Could you check a few things on this model? Use its own coordinates, in mm. A direction names the side the tool comes from. Coordinates: 2 decimals unless noted, no trailing zeros. Order: outer loops, then holes, each group sorted by start corner. A loop starts at its lowest first (then second) coordinate and runs counter-clockwise, first axis right, second up. Notation, with made-up numbers: (85, -32.75) -> (98, -32.75) arc R14 cw to (98, -25.75) -> close; hole circle Ø5 at (-31, -22.75). An arc over 180 degrees is marked (long way). Use a Markdown table: item, result. Add a question column.
1) Thinking about a two-plate mould opening in X: for faces 5 (the flat face through (2.54, 169, 0)), 6 (the flat face through (63, 75, 7.938)), 7 (the flat face through (20.4, 323.85, -0.1)), which applies, +X half, -X half, draft (parallel to the pull), parting line (faces both ways), or undercut?
2) If I drill on L1, parallel to X at y = 281, z = 2; L2, parallel to X at y = 40, z = 4 (1 decimal); L3, parallel to Y at x = 10, z = -2.5 (3 decimals), over which ranges is the centre line in solid material (lowest first)? Write a range as [from, to].
3) Will these pins go through, and if not, where does the flat tip stop? pin 1 Ø15 at (x, z) = (64, -2.5) entering from +Y; pin 2 Ø8 at (x, y) = (13, 140.5) entering from -Z (3 decimals); pin 3 Ø5 at (y, z) = (285.5, 10) entering from -X; pin 4 Ø15 at (x, y) = (63.5, 0) entering from -Z.
4) If we section it at A-A (y = 0): Write out the boundary of the cut face in (x, z) (3 decimals).
5) Which directions (+Z, -Z, +X, -X, +Y, -Y) give clear straight access to the entire face, cutting with the end or side of a thin tool? Please do faces 1 (the flat face through (12, 169, 9.525)), 2 (the flat face through (106.998, 169, 0)), 3 (the flat face through (124.46, 169, 0)), 4 (the flat face through (63, 10, 15.875)).
6) If we section it at D-D (y = 204): Write out the boundary of the cut face in (x, z) (1 decimal), plus the area to 3 significant figures.
```python
from build123d import *

# Parameters (mm, degrees)
SKETCH1_W           = 38.1
SKETCH1_H           = 38.1
SKETCH1_W_2         = 31.75
SKETCH1_H_2         = 31.75
BOSS_EXTRUDE1_DEPTH = 127
SKETCH2_W           = 19.05
SKETCH2_H           = 19.05
SKETCH2_W_2         = 15.875
SKETCH2_H_2         = 15.875
BOSS_EXTRUDE2_DEPTH = 114.3
SKETCH3_W           = 19.05
SKETCH3_H           = 19.05
SKETCH3_W_2         = 15.875
SKETCH3_H_2         = 15.875
BOSS_EXTRUDE3_DEPTH = 304.8
SKETCH4_R           = 9.525
CUT_EXTRUDE1_DEPTH  = 350.94204163


with BuildPart() as part:
    # Sketch1 → Boss-Extrude1 (new body)
    with BuildSketch(Plane(origin=(0, 0, 0), x_dir=(0, 0, -1), z_dir=(1, 0, 0))):
        Rectangle(SKETCH1_W, SKETCH1_H)
        Rectangle(SKETCH1_W_2, SKETCH1_H_2, mode=Mode.SUBTRACT)
    extrude(amount=BOSS_EXTRUDE1_DEPTH)

    # Sketch2 → Boss-Extrude2 (add)
    with BuildSketch(Plane(origin=(0, 19.05, 0), x_dir=(1, 0, 0), z_dir=(0, 1, 0))):
        with Locations((63.5, 0)):
            Rectangle(SKETCH2_W, SKETCH2_H)
        with Locations((63.5, 0)):
            Rectangle(SKETCH2_W_2, SKETCH2_H_2, mode=Mode.SUBTRACT)
    extrude(amount=BOSS_EXTRUDE2_DEPTH)

    # Sketch3 → Boss-Extrude3 (add)
    with BuildSketch(Plane(origin=(0, 19.05, 0), x_dir=(1, 0, 0), z_dir=(0, 1, 0))):
        with Locations((12.065, 0)):
            Rectangle(SKETCH3_W, SKETCH3_H)
        with Locations((12.065, 0)):
            Rectangle(SKETCH3_W_2, SKETCH3_H_2, mode=Mode.SUBTRACT)
    boss_extrude3 = extrude(amount=BOSS_EXTRUDE3_DEPTH)

    # Mirror1: Boss-Extrude3 across plane
    add(boss_extrude3.mirror(Plane.ZY.offset(-63.5)))

    # Sketch4 → Cut-Extrude1 (cut, through all)
    with BuildSketch(Plane.XY.offset(19.05)):
        with Locations((63.5, 0)):
            Circle(SKETCH4_R)
    extrude(amount=-CUT_EXTRUDE1_DEPTH, mode=Mode.SUBTRACT)


solid = part.part
```
Answer sheet:
| question | item | result |
|---|---|---|
| 1 | face 5 | -X half |
| 1 | face 6 | undercut |
| 1 | face 7 | draft |
| 2 | L1 | [2.54, 4.13], [20, 21.59], [105.41, 107], [122.87, 124.46] |
| 2 | L2 | [2.5, 4.1], [20, 21.6], [54, 55.6], [71.4, 73], [105.4, 107], [122.9, 124.5] |
| 2 | L3 | [-19.05, -15.875], [15.875, 19.05] |
| 3 | pin 1 | y = 133.35 |
| 3 | pin 2 | z = -9.525 |
| 3 | pin 3 | x = 2.54 |
| 3 | pin 4 | through |
| 4 | outline | (0, -19.05) -> (53.975, -19.05) -> (53.975, -15.875) -> (0, -15.875) -> close; (0, 15.875) -> (53.975, 15.875) -> (53.975, 19.05) -> (0, 19.05) -> close; (73.025, -19.05) -> (127, -19.05) -> (127, -15.875) -> (73.025, -15.875) -> close; (73.025, 15.875) -> (127, 15.875) -> (127, 19.05) -> (73.025, 19.05) -> close |
| 5 | face 1 | +Z, +X, -X, +Y |
| 5 | face 2 | +Y |
| 5 | face 3 | +Z, -Z, +X, +Y |
| 5 | face 4 | +X, -X |
| 6 | outline | (2.5, -9.5) -> (21.6, -9.5) -> (21.6, 9.5) -> (2.5, 9.5) -> close; (105.4, -9.5) -> (124.5, -9.5) -> (124.5, 9.5) -> (105.4, 9.5) -> close; hole (4.1, -7.9) -> (20, -7.9) -> (20, 7.9) -> (4.1, 7.9) -> close; hole (107, -7.9) -> (122.9, -7.9) -> (122.9, 7.9) -> (107, 7.9) -> close |
| 6 | area | 222 mm2 |
